from build123d import *

# Parameters (mm, degrees)
L_ANGLE_EQUAL_40X40X3_3_DEPTH = 300
SKETCH14_R                    = 4
CUT_EXTRUDE1_DEPTH            = 10


with BuildPart() as part:
    # Sketch13 → L angle (equal) 40X40X3(3) (new body)
    with BuildSketch(Plane(origin=(0, 0, 0), x_dir=(0, 0, -1), z_dir=(1, 0, 0))):
        with BuildLine():
            Line((0, 40), (0, 0))
            Line((0, 0), (40, 0))
            ThreePointArc((40, 0), (39.121320344, 2.121320344), (37, 3))
            Line((37, 3), (9, 3))
            ThreePointArc((9, 3), (4.757359313, 4.757359313), (3, 9))
            Line((3, 9), (3, 37))
            ThreePointArc((3, 37), (2.121320344, 39.121320344), (0, 40))
        make_face()
    extrude(amount=L_ANGLE_EQUAL_40X40X3_3_DEPTH)

    # Sketch14 → Cut-Extrude1 (cut)
    with BuildSketch(Plane(origin=(0, 0, 0), x_dir=(-1, 0, 0), z_dir=(0, -1, 0))):
        with Locations(Location((-280, 20, 0), (0, 0, 90))):
            Circle(SKETCH14_R)
        with Locations(Location((-20, 20, 0), (0, 0, 90))):
            Circle(SKETCH14_R)
    extrude(amount=-CUT_EXTRUDE1_DEPTH, mode=Mode.SUBTRACT)


solid = part.part
Part model, mm, in its own coordinate system. A direction names the side the tool comes from. Coordinates: 2 decimals unless noted, no trailing zeros. Loops run counter-clockwise (first coordinate to the right, second up) from the corner with the lowest first, then second, coordinate; pieces in that order, holes last. Notation, with made-up numbers: (35, 84.25) - (50, 84.25) arc R24 ccw to (50, 118.25) - close; hole circle Ø6 at (76, 21). An arc over 180 degrees is marked (long way). Write each question's results on one line, items separated by ' | '. Start each with the question number.
Q1. Slice it at A-A on x = 20. Give the cut face in (y, z), and give its area (3 significant figures).
Q2. Probe line 1 along X through (y, z) = (0.9, -20); line 2 along Z through (x, y) = (216, 27); line 3 along Y through (x, z) = (250, -26). List the from-to ranges inside material, lowest first.
Q3. Slice it at D-D on y = 34.5. Give the cut face in (x, z).
Q4. Slice it at C-C on x = 84.5. Give the cut face in (y, z).
Q5. Drop flat-ended pins along their axis: pin 1 Ø3 at (x, y) = (138, 33) entering from -Z; pin 2 Ø12 at (x, z) = (250, -19.5) entering from +Y; pin 3 Ø8 at (x, z) = (181, -33) entering from -Y. Give the stop position or say it passes through.
Q6. Which spindle directions (+Z, -Z, +X, -X, +Y, -Y) get a long thin tool onto all of the face, cutting with end or side? Do faces 4 (the flat face through (148, 23, -3)), 5 (the cylindrical face through (276.451, 1.479, -21.846)). Say none if no direction does.
Q7. Slice it at B-B on z = -20. Give the cut face in (x, y).
Q8. Two-plate mould, pull along X, no slides. Class faces 1 (the cylindrical face through (147.9, 4.711, -4.804)), 2 (the cylindrical face through (23.966, 1.479, -19.479)), 3 (the flat face through (0, 10, -2)): +X half, -X half, draft (parallel to the pull), parting line (faces both ways), or undercut.
Answer:
1) outline: (0, -40) arc R3 ccw to (3, -37) - (3, -24) - (0, -24) - close; (0, -16) - (3, -16) - (3, -9) arc R6 cw to (9, -3) - (37, -3) arc R3 ccw to (40, 0) - (0, 0) - close | area: 211 mm2
2) line 1: x = 0 to 16, 24 to 276, 284 to 300 | line 2: z = -3 to 0 | line 3: y = 0 to 3
3) outline: (0, -3) - (300, -3) - (300, 0) - (0, 0) - close
4) outline: (0, -40) arc R3 ccw to (3, -37) - (3, -9) arc R6 cw to (9, -3) - (37, -3) arc R3 ccw to (40, 0) - (0, 0) - close
5) pin 1: stops at z = -3 | pin 2: stops at y = 3 | pin 3: stops at y = 0
6) face 4: -Z, +X, -X, +Y | face 5: +Y, -Y
7) outline: (0, 0) - (16, 0) - (16, 3) - (0, 3) - close; (24, 0) - (276, 0) - (276, 3) - (24, 3) - close; (284, 0) - (300, 0) - (300, 3) - (284, 3) - close
8) face 1: draft | face 2: undercut | face 3: -X half
